Geometry check sheet. Reference: the model listing, model coordinates, mm. Coordinates: 2 decimals unless noted, no trailing zeros. Write each loop counter-clockwise with the first axis right and the second up, starting at its lowest first coordinate (ties: lowest second). Pieces come first, ordered by that corner, then holes. Notation, with made-up numbers: (16.5, 19) -> (33.5, 19) arc R6 ccw to (33.5, 24) -> close; hole circle Ø8 at (26.5, 55). An arc over 180 degrees is marked (long way). Answer in a Markdown table with one row per item. Add a question column.
Q1. Section check B-B, the plane y = 5. Count the separate pieces of the cut face and the enclosed holes in it, and give its area (3 significant figures).
Q2. Thickness scan on line 1 (Z direction, x = 687, y = 5). Record the ranges inside material, lowest first.
Q3. Section check A-A, the plane x = 373. Record the boundary of the cut face in (y, z), and give its area (3 significant figures).
```python
from build123d import *

# Parameters (mm, degrees)
SKETCH1_W               = 939.8
SKETCH1_H               = 273.05
BOSS_EXTRUDE1_DEPTH     = 6.35
CUT_EXTRUDE1_DEPTH      = 979.683127984
CUT_EXTRUDE1_DEPTH_BACK = 979.683127984
SKETCH2_W               = 44.45
SKETCH2_H               = 6.35
SKETCH2_W_2             = 88.9
SKETCH3_W               = 115.877039993
SKETCH3_H               = 273.05
CUT_EXTRUDE2_DEPTH      = 6.35


with BuildPart() as part:
    # Sketch1 → Boss-Extrude1 (new body)
    with BuildSketch(Plane(origin=(0, 0, 0), x_dir=(1, 0, 0), z_dir=(0, 1, 0))):
        with Locations((469.9, -136.525)):
            Rectangle(SKETCH1_W, SKETCH1_H)
    extrude(amount=BOSS_EXTRUDE1_DEPTH)

    # Sketch2 → Cut-Extrude1 (cut, two sides: drawn at the far end of the back side and taken through both)
    with BuildSketch(Plane(origin=(0, 6.35, 0), x_dir=(1, 0, 0), z_dir=(0, 1, 0)).offset(-CUT_EXTRUDE1_DEPTH_BACK)):
        with Locations((47.625, -29.913697199)):
            Rectangle(SKETCH2_W, SKETCH2_H)
        with Locations((130.175, -29.913697199)):
            Rectangle(SKETCH2_W, SKETCH2_H)
        with Locations((212.725, -29.913697199)):
            Rectangle(SKETCH2_W, SKETCH2_H)
        with Locations((295.275, -29.913697199)):
            Rectangle(SKETCH2_W, SKETCH2_H)
        with Locations((377.825, -29.913697199)):
            Rectangle(SKETCH2_W, SKETCH2_H)
        with Locations((460.375, -29.913697199)):
            Rectangle(SKETCH2_W, SKETCH2_H)
        with Locations((542.925, -29.913697199)):
            Rectangle(SKETCH2_W, SKETCH2_H)
        with Locations((625.475, -29.913697199)):
            Rectangle(SKETCH2_W, SKETCH2_H)
        with Locations((708.025, -29.913697199)):
            Rectangle(SKETCH2_W, SKETCH2_H)
        with Locations((790.575, -29.913697199)):
            Rectangle(SKETCH2_W, SKETCH2_H)
        with Locations((130.175, -137.863697199)):
            Rectangle(SKETCH2_W, SKETCH2_H)
        with Locations((212.725, -137.863697199)):
            Rectangle(SKETCH2_W, SKETCH2_H)
        with Locations((295.275, -137.863697199)):
            Rectangle(SKETCH2_W, SKETCH2_H)
        with Locations((377.825, -137.863697199)):
            Rectangle(SKETCH2_W, SKETCH2_H)
        with Locations((460.375, -137.863697199)):
            Rectangle(SKETCH2_W, SKETCH2_H)
        with Locations((542.925, -137.863697199)):
            Rectangle(SKETCH2_W, SKETCH2_H)
        with Locations((625.475, -137.863697199)):
            Rectangle(SKETCH2_W, SKETCH2_H)
        with Locations((708.025, -137.863697199)):
            Rectangle(SKETCH2_W, SKETCH2_H)
        with Locations((790.575, -137.863697199)):
            Rectangle(SKETCH2_W, SKETCH2_H)
        with Locations((130.175, -245.813697199)):
            Rectangle(SKETCH2_W, SKETCH2_H)
        with Locations((212.725, -245.813697199)):
            Rectangle(SKETCH2_W, SKETCH2_H)
        with Locations((295.275, -245.813697199)):
            Rectangle(SKETCH2_W, SKETCH2_H)
        with Locations((377.825, -245.813697199)):
            Rectangle(SKETCH2_W, SKETCH2_H)
        with Locations((460.375, -245.813697199)):
            Rectangle(SKETCH2_W, SKETCH2_H)
        with Locations((542.925, -245.813697199)):
            Rectangle(SKETCH2_W, SKETCH2_H)
        with Locations((625.475, -245.813697199)):
            Rectangle(SKETCH2_W, SKETCH2_H)
        with Locations((708.025, -245.813697199)):
            Rectangle(SKETCH2_W, SKETCH2_H)
        with Locations((790.575, -245.813697199)):
            Rectangle(SKETCH2_W, SKETCH2_H)
        with Locations((47.625, -137.863697199)):
            Rectangle(SKETCH2_W, SKETCH2_H)
        with Locations((47.625, -245.813697199)):
            Rectangle(SKETCH2_W, SKETCH2_H)
        with Locations((895.35, -137.863697199)):
            Rectangle(SKETCH2_W_2, SKETCH2_H)
        with Locations((895.35, -29.913697199)):
            Rectangle(SKETCH2_W_2, SKETCH2_H)
        with Locations((895.35, -245.813697199)):
            Rectangle(SKETCH2_W_2, SKETCH2_H)
    extrude(amount=CUT_EXTRUDE1_DEPTH + CUT_EXTRUDE1_DEPTH_BACK, mode=Mode.SUBTRACT)

    # Sketch3 → Cut-Extrude2 (cut)
    with BuildSketch(Plane.XZ):
        with Locations((881.861480003, 136.525)):
            Rectangle(SKETCH3_W, SKETCH3_H)
    extrude(amount=-CUT_EXTRUDE2_DEPTH, mode=Mode.SUBTRACT)


solid = part.part
```
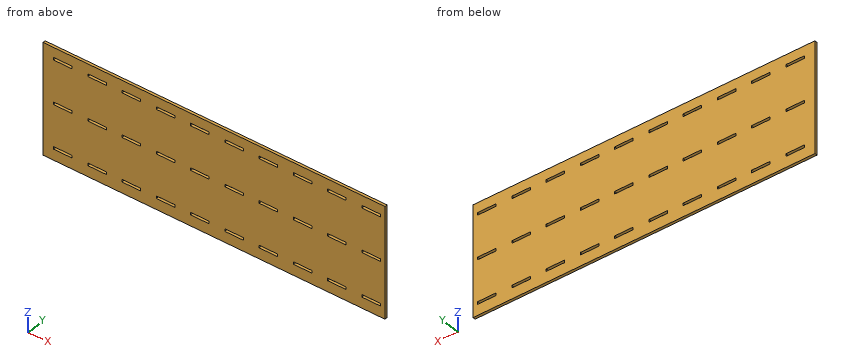
Calculated:
| question | item | result |
|---|---|---|
| 1 | separate pieces | 1 |
| 1 | enclosed holes | 30 |
| 1 | area | 217,000 mm² |
| 2 | line 1 | z = 0 to 26.74, 33.09 to 134.69, 141.04 to 242.64, 248.99 to 273.05 |
| 3 | outline | (0, 0) -> (6.35, 0) -> (6.35, 26.74) -> (0, 26.74) -> close; (0, 33.09) -> (6.35, 33.09) -> (6.35, 134.69) -> (0, 134.69) -> close; (0, 141.04) -> (6.35, 141.04) -> (6.35, 242.64) -> (0, 242.64) -> close; (0, 248.99) -> (6.35, 248.99) -> (6.35, 273.05) -> (0, 273.05) -> close |
| 3 | area | 1,610 mm² |
